Read the model definition and answer for the solid it produces. Units are mm, in the model's axes. A direction names the side the tool comes from. Coordinates: 2 decimals unless noted, no trailing zeros. Loops run counter-clockwise (first coordinate to the right, second up) from the corner with the lowest first, then second, coordinate; pieces in that order, holes last. Notation, with made-up numbers: (48, 66) - (86, 66) arc R24 cw to (86, 100) - close; hole circle Ø7 at (27, -14). An arc over 180 degrees is marked (long way). One line per item, written item: value. Start each with the question number.
from build123d import *

# Parameters (mm, degrees)
SKETCH6_R           = 24
BOSS_EXTRUDE1_DEPTH = 5
SKETCH8_R           = 1.55
CUT_EXTRUDE6_DEPTH  = 5
SKETCH10_R          = 4
BOSS_EXTRUDE2_DEPTH = 9.5
SKETCH11_R          = 3.5
CUT_EXTRUDE8_DEPTH  = 3
CUT_EXTRUDE9_DEPTH  = 8


with BuildPart() as part:
    # Sketch6 → Boss-Extrude1 (new body)
    with BuildSketch(Plane.XY):
        Circle(SKETCH6_R)
    extrude(amount=BOSS_EXTRUDE1_DEPTH)

    # Sketch8 → Cut-Extrude6 (cut)
    with BuildSketch(Plane(origin=(0, 0, 0), x_dir=(-1, 0, 0), z_dir=(0, 0, -1))):
        with Locations((0, 20)):
            Circle(SKETCH8_R)
        with Locations((14.142135624, 14.142135624)):
            Circle(SKETCH8_R)
        with Locations((20, 0)):
            Circle(SKETCH8_R)
        with Locations((14.142135624, -14.142135624)):
            Circle(SKETCH8_R)
        with Locations((0, -20)):
            Circle(SKETCH8_R)
        with Locations((-14.142135624, -14.142135624)):
            Circle(SKETCH8_R)
        with Locations((-20, 0)):
            Circle(SKETCH8_R)
        with Locations((-14.142135624, 14.142135624)):
            Circle(SKETCH8_R)
    extrude(amount=-CUT_EXTRUDE6_DEPTH, mode=Mode.SUBTRACT)

    # Sketch10 → Boss-Extrude2 (add)
    with BuildSketch(Plane.XY.offset(5)):
        Circle(SKETCH10_R)
    extrude(amount=BOSS_EXTRUDE2_DEPTH)

    # Sketch11 → Cut-Extrude8 (cut)
    with BuildSketch(Plane.XY.offset(5)):
        with Locations((0, 20)):
            Circle(SKETCH11_R)
        with Locations((14.142135624, 14.142135624)):
            Circle(SKETCH11_R)
        with Locations((20, 0)):
            Circle(SKETCH11_R)
        with Locations((14.142135624, -14.142135624)):
            Circle(SKETCH11_R)
        with Locations((0, -20)):
            Circle(SKETCH11_R)
        with Locations((-14.142135624, -14.142135624)):
            Circle(SKETCH11_R)
        with Locations((-20, 0)):
            Circle(SKETCH11_R)
        with Locations((-14.142135624, 14.142135624)):
            Circle(SKETCH11_R)
    extrude(amount=-CUT_EXTRUDE8_DEPTH, mode=Mode.SUBTRACT)

    # Sketch12 → Cut-Extrude9 (cut)
    with BuildSketch(Plane.XY.offset(14.5)):
        with BuildLine():
            Line((-1.587450787, 1.8), (1.587450787, 1.8))
            ThreePointArc((1.587450787, 1.8), (0, -2.4), (-1.587450787, 1.8))
        make_face()
    extrude(amount=-CUT_EXTRUDE9_DEPTH, mode=Mode.SUBTRACT)


solid = part.part
1) Section A-A, the plane x = 0 is taken. Determine the outline of the cut face in (y, z).
2) Section B-B, the plane y = 0 is taken. Determine the outline of the cut face in (x, z).
3) Flat-ended cylindrical pins translate along their axes: P1, Ø3, axis at y = 5, z = 8, coming from the -X side; P2, Ø5.5, axis at x = -19.5, y = 0.5, coming from the +Z side; P3, Ø10, axis at x = 19, y = -16.5, coming from the +Z side; P4, Ø1.9, axis at x = 20, y = 0, coming from the +Z side. Find the tip coordinate at first contact, or state that the pin passes through.
4) For faces 1 (the flat face through (2, 19, 2)), 2 (the cylindrical face through (0.202, -18.463, 0.986)), determine the directions among +Z, -Z, +X, -X, +Y, -Y from which every point of the face is accessible in a straight line to the end or side of a thin tool.
5) Straight lines are drawn through the part: L1, parallel to Y at x = 0, z = 1.2; L2, parallel to Y at x = 0, z = 4.15; L3, parallel to Z at x = 9, y = 20. For each, find the intervals that lie inside material, in ascending order.
6) Determine the mould class of faces 3 (the flat face through (0, 0, 0)), 4 (the cylindrical face through (-16.66, 1.05, 3.52)), 5 (the flat face through (16, -15, 2)) for opening direction Z: released by +Z, released by -Z, zero draft, split by the parting line, or undercut.
7) Section C-C, the plane x = 20 is taken. Determine the outline of the cut face in (y, z).
Answer below:
1. outline: (-24, 0) - (-21.55, 0) - (-21.55, 2) - (-23.5, 2) - (-23.5, 5) - (-24, 5) - close; (-18.45, 0) - (18.45, 0) - (18.45, 2) - (16.5, 2) - (16.5, 5) - (4, 5) - (4, 14.5) - (1.8, 14.5) - (1.8, 6.5) - (-2.4, 6.5) - (-2.4, 14.5) - (-4, 14.5) - (-4, 5) - (-16.5, 5) - (-16.5, 2) - (-18.45, 2) - close; (21.55, 0) - (24, 0) - (24, 5) - (23.5, 5) - (23.5, 2) - (21.55, 2) - close
2. outline: (-24, 0) - (-21.55, 0) - (-21.55, 2) - (-23.5, 2) - (-23.5, 5) - (-24, 5) - close; (-18.45, 0) - (18.45, 0) - (18.45, 2) - (16.5, 2) - (16.5, 5) - (4, 5) - (4, 14.5) - (2.4, 14.5) - (2.4, 6.5) - (-2.4, 6.5) - (-2.4, 14.5) - (-4, 14.5) - (-4, 5) - (-16.5, 5) - (-16.5, 2) - (-18.45, 2) - close; (21.55, 0) - (24, 0) - (24, 5) - (23.5, 5) - (23.5, 2) - (21.55, 2) - close
3. P1: x = -1.94
3. P2: z = 2
3. P3: z = 5
3. P4: through
4. face 1: +Z
4. face 2: +Z, -Z
5. L1: -24 to -21.55, -18.45 to 18.45, 21.55 to 24
5. L2: -24 to -23.5, -16.5 to 16.5, 23.5 to 24
5. L3: 0 to 5
6. face 3: released by -Z
6. face 4: zero draft
6. face 5: released by +Z
7. outline: (-13.27, 0) - (-1.55, 0) - (-1.55, 2) - (-3.5, 2) - (-3.5, 5) - (-13.27, 5) - close; (1.55, 0) - (13.27, 0) - (13.27, 5) - (3.5, 5) - (3.5, 2) - (1.55, 2) - close
